Source: CAD feature listing. Evaluate the final solid. Frame: model axes, mm. Face numbers are marked on the shaded views. Round coordinates to 2 decimals unless told otherwise and drop trailing zeros. Write each loop counter-clockwise with the first axis right and the second up, starting at its lowest first coordinate (ties: lowest second). Pieces come first, ordered by that corner, then holes. Notation, with made-up numbers: M 4,-20.75 L 29,-20.75 A22 ccw 29,-8.75 Z; hole C 17,80 d4. An arc over 180 degrees is marked long. Answer in a Markdown table with one row per item.
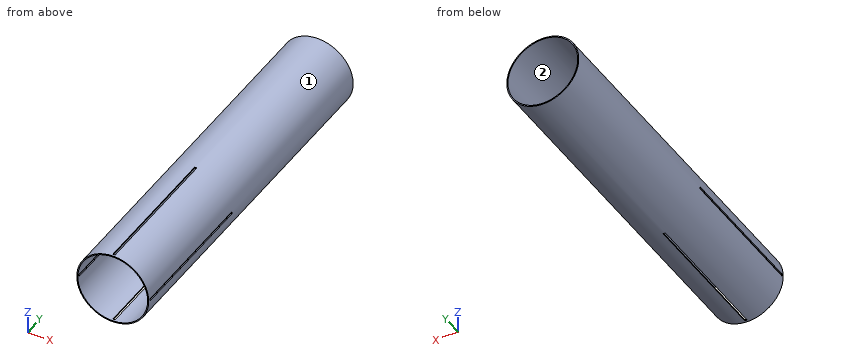
from build123d import *

# Parameters (mm, degrees)
SKETCH1_R           = 51.054
SKETCH1_R_2         = 49.53
BOSS_EXTRUDE1_DEPTH = 508
SKETCH2_W           = 3.175
SKETCH2_H           = 203.2
CUT_EXTRUDE1_DEPTH  = 52.054
CIRPATTERN1_COUNT   = 4


with BuildPart() as part:
    # Sketch1 → Boss-Extrude1 (new body)
    with BuildSketch(Plane(origin=(0, 0, 0), x_dir=(1, 0, 0), z_dir=(0, 1, 0))):
        Circle(SKETCH1_R)
        Circle(SKETCH1_R_2, mode=Mode.SUBTRACT)
    extrude(amount=BOSS_EXTRUDE1_DEPTH)

    # Sketch2 → Cut-Extrude1 (cut, through all)
    with BuildSketch(Plane.XY):
        with Locations((0, 104.775)):
            Rectangle(SKETCH2_W, SKETCH2_H)
    cut_extrude1 = extrude(amount=-CUT_EXTRUDE1_DEPTH, mode=Mode.SUBTRACT)

    # CirPattern1: Cut-Extrude1 ×4 about axis
    cirpattern1_axis = Axis((0, 0, 0), (0, 1, 0))
    for i in range(1, CIRPATTERN1_COUNT):
        add(cut_extrude1.rotate(cirpattern1_axis, i * 360 / CIRPATTERN1_COUNT), mode=Mode.SUBTRACT)


solid = part.part
Q1. Section C-C (z = -30). Return loops of the section in (x, y), and give its area (3 significant figures).
Solutions:
| item | result |
|---|---|
| outline | M -41.31,0 L -39.41,0 L -39.41,508 L -41.31,508 Z; M 39.41,0 L 41.31,0 L 41.31,508 L 39.41,508 Z |
| area | 1,930 mm2 |
Q2. Section A-A (y = 154). Return loops of the section in (x, z).
Solutions:
| item | result |
|---|---|
| outline | M -51.03,-1.59 A51.05 ccw -1.59,-51.03 L -1.59,-49.5 A49.53 cw -49.5,-1.59 Z; M -51.03,1.59 L -49.5,1.59 A49.53 cw -1.59,49.5 L -1.59,51.03 A51.05 ccw Z; M 1.59,-51.03 A51.05 ccw 51.03,-1.59 L 49.5,-1.59 A49.53 cw 1.59,-49.5 Z; M 1.59,49.5 A49.53 cw 49.5,1.59 L 51.03,1.59 A51.05 ccw 1.59,51.03 Z |
Q3. Section D-D (y = 237.5). Return loops of the section in (x, z), and give its area (3 significant figures).
Solutions:
| item | result |
|---|---|
| outline | C 0,0 d102.11; hole C 0,0 d99.06 |
| area | 482 mm2 |
Q4. Material intervals for probe 1 along Z at (x, y) = (0, 250), sorted ascending.
Solutions:
| item | result |
|---|---|
| probe 1 | z = -51.05 to -49.53, 49.53 to 51.05 |
Q5. Pull-direction query (Z, two-part tool) for the marked faces 1 and 2; classes: pulls with the +Z half, pulls with the -Z half, needs draft (parallel to the pull), parting line crosses it, or undercut.
Solutions:
| item | result |
|---|---|
| face 1 | parting line crosses it |
| face 2 | undercut |
Q6. Section B-B (x = 16). Return loops of the section in (y, z), and give its area (3 significant figures).
Solutions:
| item | result |
|---|---|
| outline | M 0,-48.48 L 508,-48.48 L 508,-46.87 L 0,-46.87 Z; M 0,46.87 L 508,46.87 L 508,48.48 L 0,48.48 Z |
| area | 1,630 mm2 |
Q7. Contact query for flat-ended pins moving along their axis: pin 1 Ø3 at (x, y) = (1.5, 79.5) entering from -Z; pin 2 Ø12 at (y, z) = (133.5, -40) entering from +X; pin 3 Ø12 at (x, y) = (14.5, 450.5) entering from -Z. Output: stop coordinate, or through.
Solutions:
| item | result |
|---|---|
| pin 1 | stops at z = -51.03 |
| pin 2 | stops at x = 38.09 |
| pin 3 | stops at z = -50.34 |
